Input: part model. Units: mm. Frame: model coordinates. A direction names the side the tool comes from. Round coordinates to 2 decimals unless told otherwise and drop trailing zeros. Loops run counter-clockwise (first coordinate to the right, second up) from the corner with the lowest first, then second, coordinate; pieces in that order, holes last. Notation, with made-up numbers: M -13.5,-29 L 30.5,-29 A6 ccw 30.5,-25 Z; hole C -27,55.25 d1. An arc over 180 degrees is marked long. Return JSON: item names as keys, results as strings. Group by question number.
1) Section C-C (y = 12). Count the separate pieces of the cut face and the enclosed holes in it, plus the area to 3 significant figures.
2) Material intervals for line 1 (Z direction, x = 13.5, y = 8.5); line 2 (X direction, y = 11, z = 15); line 3 (Z direction, x = -15, y = 3.5), sorted ascending. Write a range as from..to.
3) Section A-A (y = -15). Output: boundary loops of the cut face in (x, z), plus the area to 3 significant figures.
4) Contact query for flat-ended pins moving along their axis: P1, Ø8, axis at x = 0, z = -13.5, coming from the +Y side; P2, Ø12, axis at x = -15, z = 15, coming from the -Y side. Output: stop coordinate, or through.
5) Section B-B (x = -17). Output: boundary loops of the cut face in (y, z).
6) Section D-D (z = -5). Output: boundary loops of the cut face in (x, y), plus the area to 3 significant figures.
7) Access query for faces 3 (the face through (16, 10, -22)), 4 (the face through (-8, 5.7, 23.7)), 5 (the face through (13, 8, -10)), 6 (the face through (0, -4, -37)), 7 (the face through (0, -16, 22)). Directions: +Z, -Z, +X, -X, +Y, -Y. A direction counts if a zero-diameter tool reaches every point of the face in a straight line with its end or side. Return the directions, or none.
8) Mould query, pull axis X, two halves, no side actions, for faces 1 (the face through (0, -16, -22)), 2 (the face through (8, 5.7, 23.3)). Classes: +X half, -X half, draft (parallel to the pull), parting line (faces both ways), or undercut.
from build123d import *

# Parameters (mm, degrees)
SALIENTE_EXTRUIR1_DEPTH = 23
CORTAR_EXTRUIR1_DEPTH   = 22
CROQUIS3_W              = 10
CROQUIS3_H              = 8
CORTAR_EXTRUIR2_DEPTH   = 63.016126935


with BuildPart() as part:
    # Croquis1 → Saliente-Extruir1 (new, symmetric)
    with BuildSketch(Plane(origin=(0, 0, 0), x_dir=(0, 0, -1), z_dir=(1, 0, 0))):
        Polygon((22, -19), (37, -19), (37, 19), (-37, 19), (-37, -19), (-22, -19), (-22, -13), (22, -13), align=None)
    extrude(amount=SALIENTE_EXTRUIR1_DEPTH, both=True)

    # Croquis2 → Cortar-Extruir1 (cut)
    with BuildSketch(Plane(origin=(0, 19, 0), x_dir=(1, 0, 0), z_dir=(0, 1, 0))):
        Polygon((-8, 37), (8, 37), (8, 10), (19, 10), (19, -10), (8, -10), (8, -37), (-8, -37), (-8, -10), (-19, -10), (-19, 10), (-8, 10), align=None)
    extrude(amount=-CORTAR_EXTRUIR1_DEPTH, mode=Mode.SUBTRACT)

    # Croquis3 → Cortar-Extruir2 (cut, through all)
    with BuildSketch(Plane(origin=(23, 0, 0), x_dir=(0, 0, -1), z_dir=(1, 0, 0))):
        with Locations((27, 10)):
            Rectangle(CROQUIS3_W, CROQUIS3_H)
        with Locations((-27, 10)):
            Rectangle(CROQUIS3_W, CROQUIS3_H)
    extrude(amount=-CORTAR_EXTRUIR2_DEPTH, mode=Mode.SUBTRACT)


solid = part.part
Returned:
{
 "1": {"separate pieces": "6", "enclosed holes": "0", "area": "1,180 mm^2"},
 "2": {"line 1": "z = -37..-32, -22..-10, 10..22, 32..37", "line 2": "x = -23..-8, 8..23", "line 3": "z = -37..-10, 10..37"},
 "3": {"outline": "M -23,-37 L 23,-37 L 23,-22 L -23,-22 Z; M -23,22 L 23,22 L 23,37 L -23,37 Z", "area": "1,380 mm^2"},
 "4": {"P1": "stops at y = -3", "P2": "stops at y = -13"},
 "5": {"outline": "M -19,-37 L 19,-37 L 19,-10 L -3,-10 L -3,10 L 19,10 L 19,37 L -19,37 L -19,22 L -13,22 L -13,-22 L -19,-22 Z; hole M 6,-32 L 14,-32 L 14,-22 L 6,-22 Z; hole M 6,22 L 14,22 L 14,32 L 6,32 Z"},
 "6": {"outline": "M -23,-13 L 23,-13 L 23,19 L 19,19 L 19,-3 L -19,-3 L -19,19 L -23,19 Z", "area": "636 mm^2"},
 "7": {"face 3": "+X, -X", "face 4": "+Z, -Z, +Y", "face 5": "+Y", "face 6": "-Z, +X, -X, +Y, -Y", "face 7": "+X, -X, -Y"},
 "8": {"face 1": "draft", "face 2": "undercut"}
}
